CAD build for the part. Positions are in the model's coordinates, mm. Face numbers are marked on the shaded views. A direction names the side the tool comes from. Give positions to 0.01 mm unless a question says otherwise; leave off trailing zeros. Loops run counter-clockwise (first coordinate to the right, second up) from the corner with the lowest first, then second, coordinate; pieces in that order, holes last. Notation, with made-up numbers: M 7.5,-25 L 46.5,-25 A18 cw 46.5,6 Z; hole C 0.5,30.25 d6. An arc over 180 degrees is marked long. Answer as CSV lines item,"result".
```python
from build123d import *

# Parameters (mm, degrees)
EXTRUDE_1_DEPTH     = 7
FILLET_1_R          = 10
CHAMFER_1_SIZE      = 5
CHAMFER_2_SIZE      = 2
SKETCH_2_W          = 22.368466887
SKETCH_2_H          = 53.156625086
CUT_EXTRUDE_1_DEPTH = 100.184312104
SKETCH_3_R          = 4
CUT_EXTRUDE_2_DEPTH = 100.50128502


with BuildPart() as part:
    # Эскиз1 → Вытянуть1 (new body)
    with BuildSketch(Plane(origin=(0, 0, 0), x_dir=(0, 0, -1), z_dir=(1, 0, 0))):
        Polygon((62.822655934, -35.882923805), (59.120013374, -22.888409733), (30.956731402, -22.888409733), (30.956731402, -0.888409733), (92.539330922, -0.888409733), (92.539330922, -35.888409733), align=None)
    extrude(amount=-EXTRUDE_1_DEPTH)

    # Скругление1
    fillet_1_edges = [part.edges().sort_by_distance(p)[0] for p in [
        (-3.5, -22.888409733, -59.120013374),
    ]]
    fillet(fillet_1_edges, radius=FILLET_1_R)

    # Фаска1
    chamfer_1_edges = [part.edges().sort_by_distance(p)[0] for p in [
        (-3.5, -22.888409733, -30.956731402),
        (-3.5, -0.888409733, -30.956731402),
    ]]
    chamfer(chamfer_1_edges, length=CHAMFER_1_SIZE)

    # Фаска2
    chamfer_2_edges = [part.edges().sort_by_distance(p)[0] for p in [
        (-7, -18.388409733, -92.539330922),
    ]]
    chamfer(chamfer_2_edges, length=CHAMFER_2_SIZE)

    # Эскиз2 → Вырез-Вытянуть1 (cut, through all)
    with BuildSketch(Plane(origin=(0, -0.888409733, 0), x_dir=(-1, 0, 0), z_dir=(0, 1, 0))):
        with Locations((-10.167320296, -37.175286002)):
            Rectangle(SKETCH_2_W, SKETCH_2_H)
    extrude(amount=-CUT_EXTRUDE_1_DEPTH, mode=Mode.SUBTRACT)

    # Эскиз3 → Вырез-Вытянуть2 (cut, through all)
    with BuildSketch(Plane.ZY.offset(7)):
        with Locations((-40.076852625, -11.888409733)):
            Circle(SKETCH_3_R)
    extrude(amount=-CUT_EXTRUDE_2_DEPTH, mode=Mode.SUBTRACT)


solid = part.part
```
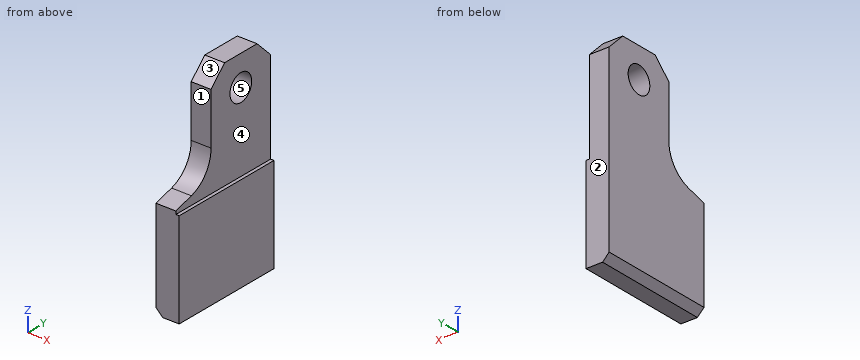
Q1. Wall check: line 1 (Z direction, x = -0.75, y = -8.5); line 2 (X direction, y = -3.5, z = -61); line 3 (Y direction, x = -5.25, z = -47). Give the ranges that are in metal, low to high. Write a range as [from, to].
Solution:
line 1,"z = [-92.54, -63.75]"
line 2,"x = [-7, -1.02]"
line 3,"y = [-22.89, -0.89]"
Q2. Mould opens along Y. For the marked faces 3, 4 and 5 say: released by +Y, released by -Y, zero draft, split by the parting line, or undercut.
Solution:
face 3,"released by -Y"
face 4,"zero draft"
face 5,"undercut"
Q3. Which spindle directions (+Z, -Z, +X, -X, +Y, -Y) get a long thin tool onto all of the face, cutting with end or side? Do the marked faces 1 and 2. Say none if no direction does.
Solution:
face 1,"+Z, +X, -X, -Y"
face 2,"+Z, -Z, +X, -X, +Y"
Q4. Cut at C-C (y = -13.5). Write the cut outline in (x, z).
Solution:
outline,"M -7,-90.54 L -5,-92.54 L 0,-92.54 L 0,-63.75 L -1.02,-63.75 L -1.02,-43.74 L -7,-43.74 Z; M -7,-36.42 L -1.02,-36.42 L -1.02,-30.96 L -7,-30.96 Z"
Q5. Cut at B-B (z = -38). Write the cut outline in (x, y).
Solution:
outline,"M -7,-22.89 L -1.02,-22.89 L -1.02,-15.31 L -7,-15.31 Z; M -7,-8.47 L -1.02,-8.47 L -1.02,-0.89 L -7,-0.89 Z"
Q6. Pin check, flat tips, straight feed: P1, Ø10, axis at y = -29.5, z = -44.5, coming from the +X side; P2, Ø6, axis at y = -8, z = -53, coming from the +X side; P3, Ø3, axis at x = -2.5, z = -46.5, coming from the -Y side; P4, Ø4, axis at x = -3, z = -64.5, coming from the -Y side. Stop position of each tip, or through.
Solution:
P1,"passes through"
P2,"stops at x = -1.02"
P3,"stops at y = -22.89"
P4,"stops at y = -35.88"
Q7. Cut at D-D (y = -3.5). Write the cut outline in (x, z).
Solution:
outline,"M -7,-90.54 L -5,-92.54 L 0,-92.54 L 0,-63.75 L -1.02,-63.75 L -1.02,-33.35 L -7,-33.35 Z"
Q8. Cut at A-A (x = -6). Write the cut outline in (y, z), and give its area (3 significant figures).
Solution:
outline,"M -35.89,-91.54 L -0.89,-91.54 L -0.89,-35.96 L -5.89,-30.96 L -17.89,-30.96 L -22.89,-35.96 L -22.89,-51.57 A10 cw -30.15,-61.19 L -35.88,-62.82 Z; hole C -11.89,-40.08 d8"
area,"1,670 mm²"
